Autodesk Inventor part; units mm, degrees
ref_plane "YZ Plane" through (0, 0, 0) normal (1, 0, 0) x (0, 1, 0)
ref_plane "XZ Plane" through (0, 0, 0) normal (0, 1, 0) x (-1, 0, 0)
ref_plane "XY Plane" through (0, 0, 0) normal (0, 0, 1) x (1, 0, 0)
sketch "Sketch1" plane through (0, 0, 0) normal (0, 0, 1) x (1, 0, 0)
  line L0 (-27, 58.4) -> (108, 58.4)
  line L1 (108, 58.4) -> (108, -10)
  line L2 (108, -10) -> (-27, -10)
  line L3 (-27, -10) -> (-27, 58.4)
  circle A0 centre (82, 0) radius 1.7
  circle A1 centre (54, 5.5) radius 1.7
  circle A2 centre (54, 32.9) radius 1.7
  circle A3 centre (75.5, 48.4) radius 1.7
  circle A4 centre (1.5, 48.4) radius 1.7
  circle A5 centre (0, 0) radius 1.7
  dimension "d63" = 82
  dimension "d64" = 48.4
  dimension "d65" = 1.5
  dimension "d66" = 15.5
  dimension "d67" = 27.4
  dimension "d68" = 48.4
  dimension "d69" = 6.5
  dimension "d70" = 74
  dimension "d71" = 5.5
  dimension "d72" = 28
  dimension "d75" = 135
  dimension "d76" = 68.4
  dimension "d77" = 10
  dimension "d78" = 27
  dimension "d79" = 3.4
  dimension "d80" = 3.4
  dimension "d81" = 3.4
  dimension "d82" = 3.4
  dimension "d83" = 3.4
  dimension "d84" = 3.4
extrude "Extrusion1" add sketch "Sketch1" along normal blind 3
sketch "Sketch2" plane through (108, -10, 0) normal (1, 0, 0) x (0, 0, -1)
  circle A0 centre (-25, 34.2) radius 10 construction
  line L0 (-3, 0) -> (-3, 68.4)
  line L1 (0, 0) -> (-3, 0)
  line L2 (-3, 0) -> (-25, 0)
  line L3 (-25, 0) -> (-25, 68.4) construction
  line L4 (-25, 68.4) -> (-3, 68.4)
  line L5 (-25, 68.4) -> (-25, 44.2)
  line L6 (-25, 0) -> (-25, 24.2)
  arc A1 (-25, 24.2) -> (-25, 44.2) centre (-25, 34.2) ccw
  point P0 (0, 10)
  point P1 (-3, 34.2)
  point P2 (-3, 34.2)
  dimension "d23" = 20
  dimension "d24" = 22
extrude "Extrusion2" add sketch "Sketch2" against normal blind 15
sketch "Sketch3" plane through (108, -10, 25) normal (0, 0, 1) x (1, 0, 0)
  circle A0 centre (-5, 5) radius 2.5
  line L0 (0, 0) -> (-15, 0)
  line L1 (0, 24.2) -> (0, 0)
  point P0 (-108, 10)
  dimension "d28" = 5
  dimension "d29" = 5
  dimension "d30" = 5
extrude "Extrusion3" cut sketch "Sketch3" against normal through all
sketch "Sketch4" plane through (0, 0, 3) normal (0, 0, 1) x (1, 0, 0)
  line L0 (-27, 58.4) -> (108, 58.4)
  line L1 (-27, 58.4) -> (-2, 58.4)
  line L2 (-2, 58.4) -> (-2, -10)
  line L3 (-2, -10) -> (-27, -10)
  line L4 (-27, -10) -> (-27, 58.4)
  point P0 (0, 0)
  point P1 (93, -10)
  dimension "d33" = 25
extrude "Extrusion4" add sketch "Sketch4" along normal blind 42
sketch "Sketch5" plane through (-2, -10, 3) normal (1, 0, 0) x (0, 0, -1)
  line L0 (0, 68.4) -> (0, 0)
  line L1 (0, 0) -> (0, 68.4)
  line L2 (0, 5) -> (-18, 5)
  line L3 (-18, 5) -> (-18, 63.4)
  line L4 (-18, 63.4) -> (0, 63.4)
  line L5 (0, 63.4) -> (0, 5)
  line L6 (3, 68.4) -> (-42, 68.4)
  point P0 (3, 10)
  point P1 (0, 8.3)
  point P2 (0, 11.7)
  point P3 (0, 23.8)
  point P4 (0, 27.2)
  point P5 (0, 51.2)
  point P6 (0, 54.6)
  point P7 (0, 56.7)
  point P8 (0, 60.1)
  point P9 (0, 56.7)
  point P10 (0, 60.1)
  point P11 (0, 8.3)
  point P12 (0, 11.7)
  dimension "d36" = 5
  dimension "d37" = 5
  dimension "d38" = 18
extrude "Extrusion5" cut sketch "Sketch5" against normal through all
sketch "Sketch6" plane through (0, 0, 3) normal (0, 0, 1) x (1, 0, 0)
  line L0 (-2, -10) -> (93, -10)
  line L1 (93, -10) -> (93, 58.4)
  line L2 (-2, -10) -> (93, -10)
  line L3 (93, -10) -> (93, -7)
  line L4 (93, -7) -> (-2, -7)
  line L5 (-2, -7) -> (-2, -10)
  line L6 (93, 58.4) -> (-2, 58.4)
  line L7 (-2, 58.4) -> (93, 58.4)
  line L8 (93, 58.4) -> (93, 55.4)
  line L9 (93, 55.4) -> (-2, 55.4)
  line L10 (-2, 55.4) -> (-2, 58.4)
  point P0 (0, 0)
  dimension "d41" = 3
  dimension "d42" = 3
extrude "Extrusion6" add sketch "Sketch6" along normal blind 42
sketch "Sketch7" plane through (108, 34.2, 25) normal (0, 0, 1) x (1, 0, 0)
  circle A0 centre (-5, 19.2) radius 2.5
  line L0 (0, 24.2) -> (-15, 24.2)
  point P0 (-108, -34.2)
  dimension "d45" = 5
  dimension "d46" = 5
  dimension "d47" = 5
extrude "Extrusion7" cut sketch "Sketch7" against normal through all
sketch "Sketch9" plane through (-2, 55.4, 3) normal (0, -1, 0) x (1, 0, 0)
  line L0 (0, 42) -> (95, 42)
  line L1 (25, 42) -> (35, 42)
  line L2 (35, 42) -> (35, 32)
  line L3 (35, 32) -> (25, 32)
  line L4 (25, 32) -> (25, 42)
  point P0 (2, -3)
  dimension "d50" = 25
  dimension "d51" = 10
  dimension "d52" = 10
extrude "Extrusion8" cut sketch "Sketch9" along normal through all both and the other way through all
sketch "Sketch10" plane through (108, -10, 0) normal (1, 0, 0) x (0, 0, -1)
  line L0 (0, 7.5) -> (0, 2.5)
  line L1 (-25, 2.5) -> (-25, 7.5)
  line L2 (0, 65.9) -> (0, 60.9)
  line L3 (-25, 60.9) -> (-25, 65.9)
  line L4 (0, 0) -> (-45, 0)
  line L5 (-20, 0) -> (-15, 0)
  line L6 (-15, 0) -> (-15, 10)
  line L7 (-15, 10) -> (-20, 10)
  line L8 (-20, 10) -> (-20, 0)
  line L9 (0, 68.4) -> (-45, 68.4)
  line L10 (-20, 68.4) -> (-15, 68.4)
  line L11 (-15, 68.4) -> (-15, 58.4)
  line L12 (-15, 58.4) -> (-20, 58.4)
  line L13 (-20, 58.4) -> (-20, 68.4)
  point P0 (0, 10)
  dimension "d55" = 5
  dimension "d56" = 10
  dimension "d57" = 5
  dimension "d58" = 10
extrude "Extrusion9" cut sketch "Sketch10" against normal blind 10
sketch "Sketch12" plane through (0, 0, 45) normal (0, 0, 1) x (1, 0, 0)
  line L0 (23, 58.4) -> (-27, 58.4)
  line L1 (-27, -10) -> (23, -10)
  line L2 (-27, 58.4) -> (-12, 58.4)
  line L3 (-12, 58.4) -> (-12, -10)
  line L4 (-12, -10) -> (-27, -10)
  line L5 (-27, -10) -> (-27, 58.4)
  line L6 (-2, -7) -> (-2, 55.4)
  point P0 (0, 0)
  dimension "d85" = 10
extrude "Extrusion10" cut sketch "Sketch12" against normal through all
sketch "Sketch13" plane through (0, 0, 45) normal (0, 0, 1) x (1, 0, 0)
  line L0 (-12, -10) -> (-12, 58.4)
  line L1 (-12, 58.4) -> (3, 58.4)
  line L2 (3, 58.4) -> (3, 43.4)
  line L3 (3, 43.4) -> (-12, 43.4)
  line L4 (-12, 43.4) -> (-12, 58.4)
  line L5 (-12, -10) -> (3, -10)
  line L6 (3, -10) -> (3, 5)
  line L7 (3, 5) -> (-12, 5)
  line L8 (-12, 5) -> (-12, -10)
  point P0 (0, 0)
  dimension "d88" = 15
  dimension "d89" = 15
  dimension "d90" = 15
  dimension "d91" = 15
extrude "Extrusion11" cut sketch "Sketch13" against normal blind 10
sketch "Sketch14" plane through (0, 0, 35) normal (0, 0, 1) x (1, 0, 0)
  circle A0 centre (-7, 53.4) radius 2.5
  circle A1 centre (-7, -5) radius 2.5
  line L0 (3, -10) -> (-12, -10)
  line L1 (-12, 58.4) -> (3, 58.4)
  line L2 (-12, 43.4) -> (-12, 58.4)
  point P0 (0, 0)
  dimension "d94" = 5
  dimension "d95" = 5
  dimension "d96" = 5
  dimension "d97" = 5
  dimension "d98" = 5
extrude "Extrusion12" cut sketch "Sketch14" against normal blind 20
sketch "Sketch15" plane through (-12, -10, 0) normal (-1, 0, 0) x (0, 0, 1)
  line L0 (30, 68.4) -> (25, 68.4)
  line L1 (25, 68.4) -> (25, 58.4)
  line L2 (25, 58.4) -> (30, 58.4)
  line L3 (30, 58.4) -> (30, 68.4)
  line L4 (25, 0) -> (45, 0)
  line L5 (30, 0) -> (25, 0)
  line L6 (25, 0) -> (25, 10)
  line L7 (25, 10) -> (30, 10)
  line L8 (30, 10) -> (30, 0)
  line L9 (0, 68.4) -> (35, 68.4)
  line L10 (35, 0) -> (35, 15)
  point P0 (0, 10)
  dimension "d101" = 5
  dimension "d102" = 10
  dimension "d103" = 10
  dimension "d104" = 5
extrude "Extrusion13" cut sketch "Sketch15" against normal blind 10
sketch "Sketch16" plane through (0, 0, 3) normal (0, 0, 1) x (1, 0, 0)
  circle A0 centre (0, 0) radius 1.7
  circle A1 centre (1.5, 48.4) radius 1.7
  circle A2 centre (54, 32.9) radius 1.7
  circle A3 centre (75.5, 48.4) radius 1.7
  circle A4 centre (54, 5.5) radius 1.7
  circle A5 centre (82, 0) radius 1.7
  circle A6 centre (75.5, 48.4) radius 4
  circle A7 centre (54, 32.9) radius 4
  circle A8 centre (54, 5.5) radius 4
  circle A9 centre (82, 0) radius 4
  circle A10 centre (0, 0) radius 1.7
  circle A11 centre (0, 0) radius 4
  circle A12 centre (1.5, 48.4) radius 4
  dimension "d107" = 8
  dimension "d108" = 8
  dimension "d109" = 8
  dimension "d110" = 8
  dimension "d111" = 8
  dimension "d112" = 8
extrude "Extrusion14" add sketch "Sketch16" along normal blind 2
properties part number "BP007" material "ABS Plastic"
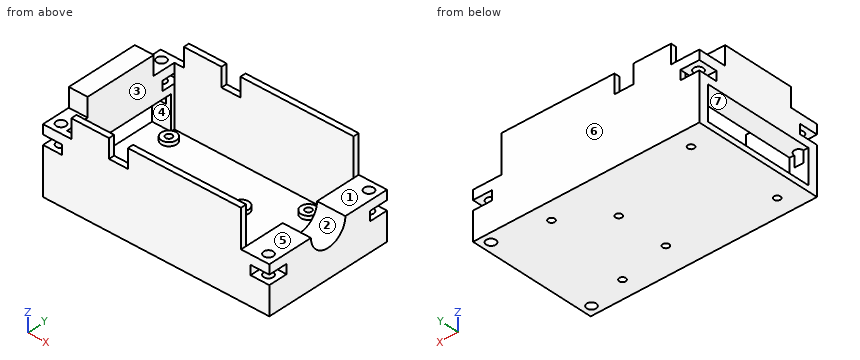
Geometry: final body of the model. Coordinates: model frame, mm. Face numbers are marked on the shaded views. A direction names the side the tool comes from. Coordinates: 2 decimals unless noted, no trailing zeros. Write each loop counter-clockwise with the first axis right and the second up, starting at its lowest first coordinate (ties: lowest second). Pieces come first, ordered by that corner, then holes. Notation, with made-up numbers: M -16.75,-7 L -12.75,-7 A32 cw -12.75,32 Z; hole C 87.5,55 d11. An arc over 180 degrees is marked long. Use CSV: the item, a comma, the result in double quotes. Start each with the question number.
1. Ray query, probe 1 along Y at (x, z) = (-7, 31.35); probe 2 along Y at (x, z) = (1.5, 20.5); probe 3 along Y at (x, z) = (82, 2). Return the intervals inside material, ascending.
2. Cut plane A-A on x = 75.5. Return the cut outline in (y, z).
3. First-contact query: P1, Ø3, axis at x = 1.5, y = 48.4, coming from the -Z side; P2, Ø2.5, axis at x = 82, y = -1, coming from the +Z side; P3, Ø8, axis at y = 1, z = 8.5, coming from the -X side; P4, Ø3, axis at x = -7.5, y = 55, coming from the +Z side. Flat tips, straight axial feed; report the tip coordinate or a pass-through.
4. Reachability of the marked faces 1, 2, 3 and 4 from +Z, -Z, +X, -X, +Y, -Y: full face, straight path, thin tool, end or side. Return the list, or none.
5. Cut plane B-B on y = 42. Return the cut outline in (x, z).
6. Cut plane C-C on z = 17. Return the cut outline in (x, y).
7. Mould query, pull axis Z, two halves, no side actions, for the marked faces 5, 6 and 7. Classes: pulls with the +Z half, pulls with the -Z half, needs draft (parallel to the pull), parting line crosses it, or undercut.
8. Cut plane D-D on y = 32.9. Return the cut outline in (x, z).
Entries:
1,probe 1,"-10 to -7.5, -2.5 to 50.9, 55.9 to 58.4"
1,probe 2,"-10 to -7, 55.4 to 58.4"
1,probe 3,"-10 to -1.7, 1.7 to 58.4"
2,outline,"M -10,0 L 46.7,0 L 46.7,5 L 44.4,5 L 44.4,3 L -7,3 L -7,45 L -10,45 Z; M 50.1,0 L 58.4,0 L 58.4,45 L 55.4,45 L 55.4,3 L 52.4,3 L 52.4,5 L 50.1,5 Z"
3,P1,"through"
3,P2,"z = 5"
3,P3,"x = -4"
3,P4,"z = 35"
4,face 1,"+Z, +X, +Y, -Y"
4,face 2,"+Z, +X"
4,face 3,"+Z"
4,face 4,"-X"
5,outline,"M -12,0 L 108,0 L 108,25 L 93,25 L 93,3 L -12,3 Z; M -12,21 L -2,21 L -2,45 L -12,45 Z"
6,outline,"M -12,-10 L 98,-10 L 98,0 L 108,0 L 108,18.2 L 93,18.2 L 93,-7 L -2,-7 L -2,-5 L -4.5,-5 A2.5 cw -9.5,-5 L -12,-5 Z; M -12,53.4 L -9.5,53.4 A2.5 cw -4.5,53.4 L -2,53.4 L -2,55.4 L 93,55.4 L 93,30.2 L 108,30.2 L 108,48.4 L 98,48.4 L 98,58.4 L -12,58.4 Z"
7,face 5,"pulls with the +Z half"
7,face 6,"needs draft"
7,face 7,"undercut"
8,outline,"M -12,0 L 52.3,0 L 52.3,5 L 50,5 L 50,3 L -12,3 Z; M -12,21 L -2,21 L -2,45 L -12,45 Z; M 55.7,0 L 108,0 L 108,20.07 L 93,20.07 L 93,3 L 58,3 L 58,5 L 55.7,5 Z"
